Geometry check sheet. Reference: the model listing, model coordinates, mm. A direction names the side the tool comes from. Give positions to 0.01 mm unless a question says otherwise; leave off trailing zeros. Write each loop counter-clockwise with the first axis right and the second up, starting at its lowest first coordinate (ties: lowest second). Pieces come first, ordered by that corner, then holes. Notation, with made-up numbers: M -27.75,79 L -20.75,79 A23 cw -20.75,112 Z; hole C -16,37.25 d6. An arc over 180 degrees is marked long. Use one line per item in the form item = value. Start each with the question number.
```python
from build123d import *

# Parameters (mm, degrees)
F1_DEPTH = 50.8
F2_R     = 5.08
F3_R     = 9.398
F4_DEPTH = 5.08


with BuildPart() as f1:
    # F0 (on Front) → F1 (new body)
    with BuildSketch(Plane.XZ):
        Polygon((0, -15.438433), (0, 0), (50.8, 0), (50.8, -15.438433), (57.15, -15.438433), (57.15, 9.961567), (50.8, 9.961567), (0, 9.961567), (-6.35, 9.961567), (-63.5, 9.961567), (-63.5, -0.038433), (-6.35, -0.003843), (-6.35, -15.438433), align=None)
    extrude(amount=-F1_DEPTH)

    # F2
    f2_edges = [f1.edges().sort_by_distance(p)[0] for p in [
        (57.15, 25.4, 9.961567),
    ]]
    fillet(f2_edges, radius=F2_R)

    # F3 (on face) → F4 (cut)
    with BuildSketch(Plane(origin=(0, 0, 0), x_dir=(1, 0, 0), z_dir=(0, 0, -1))):
        with Locations((25.4, -25.4)):
            Circle(F3_R)
    extrude(amount=-F4_DEPTH, mode=Mode.SUBTRACT)


solid = f1.part
```
(1) Depth check by flat-ended pin: pin 1 (12 mm diameter, centred on x = 30, y = 14.5, fed in from -Z); pin 2 (7.5 mm diameter, centred on y = 23, z = -9, fed in from -X); pin 3 (3 mm diameter, centred on x = 20.5, y = 29.5, fed in from -Z). Enter the tip coordinate at first touch or a pass-through.
(2) Sectioned sample at D-D, the plane y = 25.4. Record the boundary of the cut face in (x, z), plus the area to 3 significant figures.
(3) Sectioned sample at C-C, the plane x = 25.4. Record the boundary of the cut face in (y, z).
(4) Thickness scan on probe 1 along X at (y, z) = (43, -4.25); probe 2 along Y at (x, z) = (25.4, 2.2); probe 3 along X at (y, z) = (25.4, 2.4). Record the ranges inside material, lowest first. Write a range as [from, to].
(5) Sectioned sample at B-B, the plane z = -6.5. Record the boundary of the cut face in (x, y), plus the area to 3 significant figures.
(6) Sectioned sample at A-A, the plane y = 5.5. Record the boundary of the cut face in (x, z), plus the area to 3 significant figures.
(7) Tool access check on faces 4 (the flat face through (-5, 25, 9.962)), 5 (the flat face through (36, 25, 0)), 6 (the flat face through (-6.35, 25, -8)), 7 (the cylindrical face through (23.363, 34.575, 2.504)). Record the directions out of +Z, -Z, +X, -X, +Y, -Y that give a thin tool (end or side, any length) a straight path to the whole face; none if there is none.
(8) Draft check along Y on faces 1 (the flat face through (-4, 50.8, 3)), 2 (the flat face through (25, 25, 5.08)), 3 (the flat face through (57.15, 25, -5)). Enter one of: released by +Y, released by -Y, zero draft, split by the parting line, or undercut.
Numbers:
q1.pin_1 = 0
q1.pin_2 = -6.35
q1.pin_3 = 5.08
q2.outline = M -63.5,-0.04 L -6.35,0 L -6.35,-15.44 L 0,-15.44 L 0,0 L 16,0 L 16,5.08 L 34.8,5.08 L 34.8,0 L 50.8,0 L 50.8,-15.44 L 57.15,-15.44 L 57.15,4.88 A5.08 ccw 52.07,9.96 L -63.5,9.96 Z
q2.area = 1,300 mm2
q3.outline = M 0,0 L 16,0 L 16,5.08 L 34.8,5.08 L 34.8,0 L 50.8,0 L 50.8,9.96 L 0,9.96 Z
q4.probe_1 = [-6.35, 0], [50.8, 57.15]
q4.probe_2 = [0, 16], [34.8, 50.8]
q4.probe_3 = [-63.5, 16], [34.8, 57.15]
q5.outline = M -6.35,0 L 0,0 L 0,50.8 L -6.35,50.8 Z; M 50.8,0 L 57.15,0 L 57.15,50.8 L 50.8,50.8 Z
q5.area = 645 mm2
q6.outline = M -63.5,-0.04 L -6.35,0 L -6.35,-15.44 L 0,-15.44 L 0,0 L 50.8,0 L 50.8,-15.44 L 57.15,-15.44 L 57.15,4.88 A5.08 ccw 52.07,9.96 L -63.5,9.96 Z
q6.area = 1,390 mm2
q7.face_4 = +Z, +X, -X, +Y, -Y
q7.face_5 = -Z, +Y, -Y
q7.face_6 = -Z, -X, +Y, -Y
q7.face_7 = -Z
q8.face_1 = released by +Y
q8.face_2 = undercut
q8.face_3 = zero draft
